Work out the finished part from the listing and answer in its coordinate system (mm). Coordinates: 2 decimals unless noted, no trailing zeros. Order: outer loops, then holes, each group sorted by start corner. A loop starts at its lowest first (then second) coordinate and runs counter-clockwise, first axis right, second up. Notation, with made-up numbers: M 6.25,3.25 L 34.25,3.25 A13 cw 34.25,16.25 Z; hole C -0.5,17.25 d8. An arc over 180 degrees is marked long. Write item = value, one per line. Start each with the question number.
Q1. Find section C-C on x = 19. Give the vertices of the cut face in (y, z) (3 decimals), and give its area (3 significant figures).
Q2. This flat-tipped pin is pushed along its axis until it touches: P1, Ø1.5, axis at y = -0.5, z = -15.5, coming from the +X side. Where does it stop, or does it pass through?
Q3. Find section A-A on x = 80.5. Give the vertices of the cut face in (y, z) (3 decimals), and give its area (3 significant figures).
Q4. Find section D-D on x = -57.5. Give the vertices of the cut face in (y, z) (3 decimals), and give its area (3 significant figures).
Q5. Straight lines are drawn through the part: line 1 along X through (y, z) = (-2, 12.5); line 2 along Z through (x, y) = (96.5, -1.25); line 3 along Z through (x, y) = (-27.5, 2.5). For each, find the intervals that lie inside material, in ascending order.
Q6. Find section B-B on y = 2. Give the number of separate pieces and of enclosed holes in the cut face, and give its area (3 significant figures).
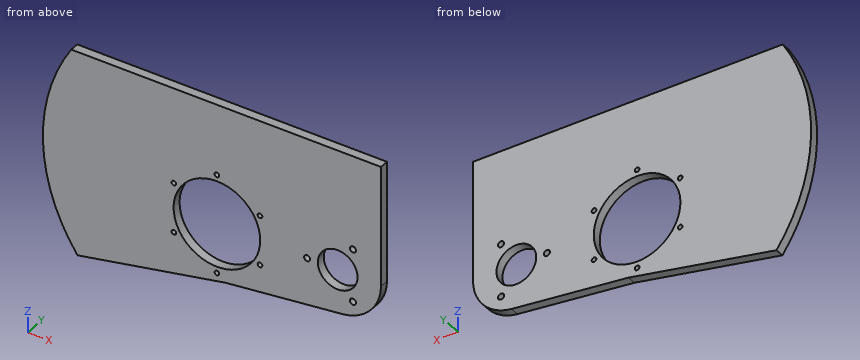
```python
from build123d import *

# Parameters (mm, degrees)
SKETCH1_R             = 30.5
SKETCH1_R_2           = 14
BOSS_EXTRUDE1_DEPTH   = 3.175
M4X0_7_TAPPED_HOLE1_D = 3.3
M4_CLEARANCE_HOLE1_D  = 4.3


with BuildPart() as part:
    # Sketch1 → Boss-Extrude1 (new, symmetric)
    with BuildSketch(Plane(origin=(0, 0, 0), x_dir=(1, 0, 0), z_dir=(0, 1, 0))):
        with BuildLine():
            Line((6.094023378, 39.566801218), (-98.107084352, 60))
            ThreePointArc((-98.107084352, 60), (-122.409547316, -11.830277132), (-102.5, -85))
            Line((-102.5, -85), (115.5, -85))
            Line((115.5, -85), (115.5, 0))
            ThreePointArc((115.5, 0), (107.74004307, 20.325856468), (88.408823529, 30.308908297))
            Line((88.408823529, 30.308908297), (6.094023378, 39.566801218))
        make_face()
        with Locations(Location((0, 0, 0), (0, 0, 270))):
            Circle(SKETCH1_R, mode=Mode.SUBTRACT)
        with Locations(Location((85, 0, 0), (0, 0, 270))):
            Circle(SKETCH1_R_2, mode=Mode.SUBTRACT)
    extrude(amount=BOSS_EXTRUDE1_DEPTH, both=True)

    # M4x0.7 Tapped Hole1 (through all)
    with Locations(Plane(origin=(0, 3.175, 0), x_dir=(1, 0, 0), z_dir=(0, 1, 0))):
        with Locations((-30.310889132, 17.5), (0, 35), (30.310889132, 17.5), (30.310889132, -17.5), (0, -35), (-30.310889132, -17.5)):
            Hole(M4X0_7_TAPPED_HOLE1_D / 2)

    # M4 Clearance Hole1 (through all)
    with Locations(Plane(origin=(0, 3.175, 0), x_dir=(1, 0, 0), z_dir=(0, 1, 0))):
        with Locations((63.5, 0), (95.75, 18.619546181), (95.75, -18.619546181)):
            Hole(M4_CLEARANCE_HOLE1_D / 2)


solid = part.part
```
Findings below:
q1.outline = M -3.175,-38.115 L 3.175,-38.115 L 3.175,-23.859 L -3.175,-23.859 Z; M -3.175,23.859 L 3.175,23.859 L 3.175,85 L -3.175,85 Z
q1.area = 479 mm^2
q2.P1 = 111.7
q3.outline = M -3.175,-31.198 L 3.175,-31.198 L 3.175,-13.257 L -3.175,-13.257 Z; M -3.175,13.257 L 3.175,13.257 L 3.175,85 L -3.175,85 Z
q3.area = 569 mm^2
q4.outline = M -3.175,-52.037 L 3.175,-52.037 L 3.175,85 L -3.175,85 Z
q4.area = 870 mm^2
q5.line_1 = -122.43 to -27.82, 27.82 to 78.7, 91.3 to 115.5
q5.line_2 = -28.25 to -20.63, -16.6 to -7.98, 7.98 to 16.6, 20.63 to 85
q5.line_3 = -46.15 to -13.19, 13.19 to 85
q6.separate_pieces = 1
q6.enclosed_holes = 11
q6.area = 25,700 mm^2
